Work out the finished part from the listing and answer in its coordinate system (mm). Round coordinates to 2 decimals unless told otherwise and drop trailing zeros. Loops run counter-clockwise (first coordinate to the right, second up) from the corner with the lowest first, then second, coordinate; pieces in that order, holes last.
Autodesk Inventor part; units mm, degrees
ref_plane "YZ Plane" through (0, 0, 0) normal (1, 0, 0) x (0, 1, 0)
ref_plane "XZ Plane" through (0, 0, 0) normal (0, 1, 0) x (-1, 0, 0)
ref_plane "XY Plane" through (0, 0, 0) normal (0, 0, 1) x (1, 0, 0)
sketch "Sketch1" plane through (0, 0, 0) normal (0, 1, 0) x (-1, 0, 0)
  line L0 (0, 0) -> (17.5, 0)
  line L1 (17.5, 0) -> (17.5, -43)
  line L2 (17.5, -43) -> (0, -43)
  line L3 (0, -43) -> (0, 0)
  dimension "d0" = 43
  dimension "d1" = 17.5
extrude "Extrusion1" add sketch "Sketch1" along normal blind 1.6
sketch "Sketch2" plane through (0, 1.6, 0) normal (0, 1, 0) x (1, 0, 0)
  line L0 (-17.5, 0) -> (0, 0)
  line L1 (-8.75, 0) -> (-8.75, 8.3818) construction
  line L2 (-5, 7.6) -> (-12.5, 7.6)
  line L3 (-12.5, 7.6) -> (-12.5, -1.6)
  line L4 (-12.5, -1.6) -> (-5, -1.6)
  line L5 (-5, -1.6) -> (-5, 7.6)
  line L6 (-5, 7.6) -> (-12.5, -1.6) construction
  line L7 (-12.5, 7.6) -> (-5, -1.6) construction
  point P0 (-8.75, 3)
  dimension "d4" = 9.2
  dimension "d5" = 7.5
  dimension "d6" = 1.6
extrude "Extrusion2" add sketch "Sketch2" along normal blind 3.8
properties part number "Arduino"
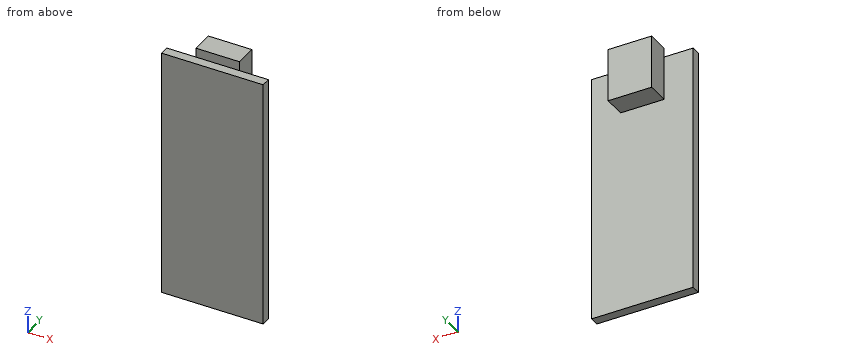
1. Consider probe 1 along Y at (x, z) = (-2.5, -1.5); probe 2 along Y at (x, z) = (-12.25, 0.5); probe 3 along Z at (x, y) = (-2.75, 0.3). Determine where each line is inside the solid, lowest interval first.
Answer key:
probe 1: y = 0 to 1.6
probe 2: y = 1.6 to 5.4
probe 3: z = -43 to 0
2. Find section A-A (z = -6). Write down the section's boundary in (x, y), then the cut area to 3 significant figures.
Answer key:
outline: (-17.5, 0) - (0, 0) - (0, 1.6) - (-5, 1.6) - (-5, 5.4) - (-12.5, 5.4) - (-12.5, 1.6) - (-17.5, 1.6) - close
area: 56.5 mm2
3. Find section D-D (z = -15). Write down the section's boundary in (x, y), then the cut area to 3 significant figures.
Answer key:
outline: (-17.5, 0) - (0, 0) - (0, 1.6) - (-17.5, 1.6) - close
area: 28.0 mm2
4. Find section B-B (x = -6). Write down the section's boundary in (y, z).
Answer key:
outline: (0, -43) - (1.6, -43) - (1.6, -7.6) - (5.4, -7.6) - (5.4, 1.6) - (1.6, 1.6) - (1.6, 0) - (0, 0) - close
5. Find section C-C (y = 3.75). Write down the section's boundary in (x, z).
Answer key:
outline: (-12.5, -7.6) - (-5, -7.6) - (-5, 1.6) - (-12.5, 1.6) - close
6. Given pin 1 (3 mm diameter, centred on x = -10, y = 3.5, fed in from -Z); pin 2 (1.1 mm diameter, centred on y = 3.5, z = -3, fed in from +X); pin 3 (1 mm diameter, centred on x = -13.5, y = 1.5, fed in from +Z), each flat-ended and moving along its own axis, determine where each tip first touches the part or whether it passes through.
Answer key:
pin 1: stops at z = -7.6
pin 2: stops at x = -5
pin 3: stops at z = 0
